Autodesk Inventor part; units mm, degrees
ref_plane "YZ Plane" through (0, 0, 0) normal (1, 0, 0) x (0, 1, 0)
ref_plane "XZ Plane" through (0, 0, 0) normal (0, 1, 0) x (-1, 0, 0)
ref_plane "XY Plane" through (0, 0, 0) normal (0, 0, 1) x (1, 0, 0)
ref_plane "Work Plane1" through (0, 0, -6) normal (0, 0, 1) x (1, 0, 0)
sketch "Sketch2" plane through (0, 0, -6) normal (0, 0, 1) x (1, 0, 0)
  line L0 (-0.1721, 1.3319) -> (-0.1721, -0.6681)
  line L1 (-0.1721, -0.6681) -> (-1.1721, -0.6681)
  line L2 (-1.1721, -0.6681) -> (-1.1721, -1.1681)
  line L3 (-1.1721, -1.1681) -> (0.1026, -1.1681)
  line L4 (0.1026, -1.1681) -> (1.1279, 1.3319)
  line L5 (-0.1721, 1.3319) -> (1.1279, 1.3319)
  line L6 (21.2279, 14.4069) -> (21.2279, 6.7069)
  line L7 (22.1279, 8.9819) -> (22.1279, 10.9819)
  line L8 (-1.5666, 1.1673) -> (16.9443, 1.1673)
  arc A0 (16.9443, 1.1673) -> (19.3523, 3.5752) centre (16.9443, 3.5752) ccw
  line L9 (19.3523, 3.5752) -> (19.3523, 9.9819)
  line L10 (20.5023, 9.9819) -> (20.5023, 3.5752)
  arc A1 (16.9443, 0.0173) -> (20.5023, 3.5752) centre (16.9443, 3.5752) ccw
  line L11 (16.9443, 0.0173) -> (-1.5666, 0.0173)
  line L12 (-1.5666, 0.0173) -> (-1.5666, 1.1673)
  line L13 (20.5023, 9.9819) -> (19.3523, 9.9819)
  line L14 (-1.5666, 18.7964) -> (16.9443, 18.7964)
  arc A2 (19.3523, 16.3885) -> (16.9443, 18.7964) centre (16.9443, 16.3885) ccw
  line L15 (19.3523, 16.3885) -> (19.3523, 9.9819)
  line L16 (20.5023, 9.9819) -> (20.5023, 16.3885)
  arc A3 (20.5023, 16.3885) -> (16.9443, 19.9464) centre (16.9443, 16.3885) ccw
  line L17 (16.9443, 19.9464) -> (-1.5666, 19.9464)
  line L18 (-1.5666, 19.9464) -> (-1.5666, 18.7964)
  point P0 (0, 0)
  point P1 (22.1279, 9.9819)
  dimension "d1" = 1.15
  dimension "d2" = 0.7257
extrude "Extrusion1" add sketch "Sketch2" along normal mid plane 8.3 contours L8 L4 L11 L0 | L0 L11 L12 L8 | L8 A0 L9 L13 L10 A1 L11 L4 | L15 A2 L14 L18 L17 A3 L16 L13
sketch "Sketch3" plane through (20.5023, 3.5752, -1.85) normal (1, 0, 0) x (0, 0, -1)
  line L0 (1.1743, 2.6316) -> (7.1257, 2.6316)
  line L1 (1.1743, 2.6316) -> (7.1257, 2.6316)
  arc A0 (0.838, 2.7615) -> (1.1743, 2.6316) centre (1.1743, 3.1316) ccw
  arc A1 (7.462, 2.7615) -> (0.838, 2.7615) centre (4.15, 6.4066) ccw
  arc A2 (7.1257, 2.6316) -> (7.462, 2.7615) centre (7.1257, 3.1316) ccw
  line L2 (1.1743, 2.6316) -> (7.1257, 2.6316)
  arc A3 (-1.1794, 0.5412) -> (1.1743, -0.3684) centre (1.1743, 3.1316) ccw
  arc A4 (9.4794, 0.5412) -> (-1.1794, 0.5412) centre (4.15, 6.4066) ccw
  arc A5 (7.1257, -0.3684) -> (9.4794, 0.5412) centre (7.1257, 3.1316) ccw
  line L3 (7.1257, -0.3684) -> (1.1743, -0.3684)
  point P0 (-1.85, -3.5752)
  dimension "d5" = 3
extrude "Extrusion2" add sketch "Sketch3" against normal blind 1.15
sketch "Sketch4" plane through (20.5023, 9.9819, -6) normal (1, 0, 0) x (0, 0, -1)
  line L0 (-2.9757, -3.775) -> (2.9757, -3.775)
  line L1 (-2.9757, -3.775) -> (2.9757, -3.775)
  arc A0 (-3.312, -3.6451) -> (-2.9757, -3.775) centre (-2.9757, -3.275) ccw
  arc A1 (3.312, -3.6451) -> (-3.312, -3.6451) centre (0, 0) ccw
  arc A2 (2.9757, -3.775) -> (3.312, -3.6451) centre (2.9757, -3.275) ccw
  point P0 (-6, -9.9819)
extrude "Extrusion3" cut sketch "Sketch4" against normal blind 1.5
fillet "Fillet1" radius 0.5 4 edges at (19.9253, 3.4097, -1.85) (19.9253, 3.4097, -10.15) (19.9189, 16.7334, -10.15) (19.9189, 16.7334, -1.85)
sketch "Sketch5" plane through (-1.5666, 0.0173, -1.85) normal (0, -1, 0) x (1, 0, 0)
  line L0 (1.3946, -7.15) -> (1.3946, -1.15)
  line L1 (1.3946, -1.15) -> (1.3946, -7.15)
  line L2 (1.6693, -1.15) -> (2.6946, -1.15)
  line L3 (1.6693, -1.15) -> (1.6693, -7.15)
  line L4 (1.6693, -7.15) -> (2.6946, -7.15)
  line L5 (2.6946, -1.15) -> (2.6946, -7.15)
  line L6 (1.1946, -7.25) -> (5.6946, -7.25)
  line L7 (5.6946, -7.25) -> (5.6946, -1.05)
  line L8 (5.6946, -1.05) -> (1.1946, -1.05)
  line L9 (1.1946, -1.05) -> (1.1946, -7.25)
  point P0 (1.5666, 1.85)
  dimension "d12" = 0.1
  dimension "d13" = 0.1
  dimension "d14" = 3
  dimension "d15" = 0.2
extrude "Extrusion4" cut sketch "Sketch5" against normal blind 22.75 contours L2 L5 L4 L3 | L9 L8 L7 L6
sketch "Sketch6" plane through (-1.5666, 0.0173, -1.85) normal (0, -1, 0) x (1, 0, 0)
  line L0 (-0.3816, -10.25) -> (8.1946, -10.25)
  line L1 (8.6946, -9.75) -> (8.6946, 1.45)
  line L2 (8.1946, 1.95) -> (-0.3799, 1.95)
  line L3 (-0.8749, -9.8319) -> (-0.9996, -9.0812)
  line L4 (-1.0196, 0.6268) -> (-0.8734, 1.5299)
  line L5 (1.1946, -1.05) -> (5.6946, -1.05)
  line L6 (5.6946, -7.25) -> (1.1946, -7.25)
  line L7 (5.6946, -1.05) -> (5.6946, -7.25)
  line L8 (1.1946, -7.25) -> (1.1946, -1.05)
  arc A0 (-1.0196, 0.6268) -> (-0.9996, -9.0812) centre (28.5951, -4.1661) ccw
  arc A1 (-0.8749, -9.8319) -> (-0.3816, -10.25) centre (-0.3816, -9.75) ccw
  arc A2 (-0.3799, 1.95) -> (-0.8734, 1.5299) centre (-0.3799, 1.45) ccw
  arc A3 (8.6946, 1.45) -> (8.1946, 1.95) centre (8.1946, 1.45) ccw
  arc A4 (8.1946, -10.25) -> (8.6946, -9.75) centre (8.1946, -9.75) ccw
  point P0 (1.5666, 1.85)
  point P1 (-0.8054, -10.25)
  point P2 (-0.8054, 1.95)
  point P3 (-1.8054, -4.2289)
  dimension "d18" = 3
  dimension "d19" = 3
  dimension "d20" = 3
  dimension "d21" = 3
  dimension "d22" = 2
  dimension "d23" = 30
  dimension "d24" = 0.5
extrude "Extrusion5" add sketch "Sketch6" against normal blind 1.15
sketch "Sketch7" plane through (-1.5666, 19.9464, -1.85) normal (0, 1, 0) x (1, 0, 0)
  line L0 (5.6946, 1.05) -> (5.6946, 7.25)
  line L1 (5.6946, 7.25) -> (1.1946, 7.25)
  line L2 (1.1946, 7.25) -> (1.1946, 1.05)
  line L3 (1.1946, 1.05) -> (5.6946, 1.05)
  line L4 (18.5109, 8.3) -> (8.6946, 8.3)
  line L5 (18.5109, 8.3) -> (18.5109, 0)
  line L6 (8.6946, 0) -> (18.5109, 0)
  line L7 (8.6946, -1.45) -> (8.6946, 0)
  arc A0 (8.1946, -1.95) -> (8.6946, -1.45) centre (8.1946, -1.45) ccw
  line L8 (-0.3799, -1.95) -> (8.1946, -1.95)
  arc A1 (-0.8734, -1.5299) -> (-0.3799, -1.95) centre (-0.3799, -1.45) ccw
  line L9 (-1.0196, -0.6268) -> (-0.8734, -1.5299)
  arc A2 (-0.9996, 9.0812) -> (-1.0196, -0.6268) centre (28.5951, 4.1661) ccw
  line L10 (-0.8749, 9.8319) -> (-0.9996, 9.0812)
  arc A3 (-0.3816, 10.25) -> (-0.8749, 9.8319) centre (-0.3816, 9.75) ccw
  line L11 (8.1946, 10.25) -> (-0.3816, 10.25)
  arc A4 (8.6946, 9.75) -> (8.1946, 10.25) centre (8.1946, 9.75) ccw
  line L12 (8.6946, 8.3) -> (8.6946, 9.75)
  point P0 (1.5666, -1.85)
extrude "Extrusion6" add sketch "Sketch7" against normal blind 1.15
fillet "Fillet2" radius 0.5 4 edges at (7.1279, 19.3714, -1.85) (7.1279, 0.5923, -1.85) (7.1279, 19.3714, -10.15) (7.1279, 0.5923, -10.15)
properties part number "Part3 - Gearbox" material "Glass"
Part model, mm, in its own coordinate system. A direction names the side the tool comes from. Coordinates: 2 decimals unless noted, no trailing zeros. Order: outer loops, then holes, each group sorted by start corner. A loop starts at its lowest first (then second) coordinate and runs counter-clockwise, first axis right, second up.
(1) Pull direction Y, two halves, no side cores. Call faces 1 (the face through (19.935, 3.837, -10.979)), 2 (the face through (4.128, 19, -6)), 3 (the face through (7, 19.946, -6)), 4 (the face through (19.94, 6.81, -2.23)): pulls with the +Y half, pulls with the -Y half, needs draft (parallel to the pull), parting line crosses it, or undercut.
Check sheet entries:
face 1: pulls with the -Y half
face 2: needs draft
face 3: pulls with the +Y half
face 4: undercut
(2) Tool access for faces 5 (the face through (2, 19, -9.1)), 6 (the face through (7.128, 19, -1)), 7 (the face through (7.128, 19, -11)): list every direction of +Z, -Z, +X, -X, +Y, -Y with a clear straight run to the whole face (end or side of a thin tool).
Check sheet entries:
face 5: +Y, -Y
face 6: +Z, +X, +Y, -Y
face 7: -Z, +X, +Y, -Y
(3) Probe L1, parallel to Y at x = 11, z = -4.75; L2, parallel to X at y = 4.75, z = -7; L3, parallel to X at y = 19, z = -8. List the from-to ranges inside material, lowest first.
Check sheet entries:
L1: y = 0.02 to 1.17, 18.8 to 19.95
L2: x = 19.35 to 20.5
L3: x = -2.91 to -0.37, 4.13 to 19.36
(4) Slice it at C-C, the plane z = -7.25. State how many separate pieces and enclosed holes the cut face has, and give its area (3 significant figures).
Check sheet entries:
separate pieces: 4
enclosed holes: 0
area: 51.2 mm2
(5) Pin check, flat tips, straight feed: pin 1 Ø1.3 at (x, y) = (4, 19.5) entering from -Z; pin 2 Ø0.9 at (x, y) = (2, 19) entering from +Z; pin 3 Ø1.8 at (x, y) = (16, 17.5) entering from -Z; pin 4 Ø0.9 at (y, z) = (19.5, -5.5) entering from +X. Stop position of each tip, or through.
Check sheet entries:
pin 1: stops at z = -12.1
pin 2: stops at z = 0.1
pin 3: passes through
pin 4: stops at x = 19.31
(6) Slice it at B-B, the plane y = 12. Write the cut outline in (x, z), and give its area (3 significant figures).
Check sheet entries:
outline: (19.35, -13.66) - (20.5, -13.66) - (20.5, -10.49) - (19.35, -10.49) - close; (19.35, -1.51) - (20.5, -1.51) - (20.5, 1.66) - (19.35, 1.66) - close
area: 7.29 mm2
(7) Slice it at A-A, the plane x = 13.5. Write the cut outline in (y, z).
Check sheet entries:
outline: (0.02, -10.15) - (1.17, -10.15) - (1.17, -1.85) - (0.02, -1.85) - close; (18.8, -10.15) - (19.95, -10.15) - (19.95, -1.85) - (18.8, -1.85) - close
(8) Slice it at D-D, the plane y = 16. Write the cut outline in (x, z).
Check sheet entries:
outline: (19.35, -11.16) - (20.5, -11.16) - (20.5, -0.84) - (19.35, -0.84) - close
